Verification items for the finished model (mm, model axes). A direction names the side the tool comes from. Give positions to 0.01 mm unless a question says otherwise; leave off trailing zeros. Loops run counter-clockwise (first coordinate to the right, second up) from the corner with the lowest first, then second, coordinate; pieces in that order, holes last. Notation, with made-up numbers: (61.5, 19.25) - (92.5, 19.25) arc R29 ccw to (92.5, 39.25) - close; hole circle Ø11 at (-5, 1). An arc over 180 degrees is marked (long way). One line per item, written item: value. Start each with the question number.
1. Sectioned sample at B-B (y = 18). Record the cut outline in (x, z), plus the area to 3 significant figures.
2. Scan lines: L1, parallel to Z at x = 12, y = -33; L2, parallel to X at y = 19, z = 3.5; L3, parallel to Y at x = -8, z = -10. Record each from-to range of solid material in increasing order. Write a range as [from, to].
3. Access from +Z, -Z, +X, -X, +Y, -Y to the whole of each face (thin tool, end or side, straight path). Record for faces 5 (the cylindrical face through (9.295, 26.827, 0.35)), 6 (the flat face through (12, -25, -17)).
4. Gauge pin test, flat ends, axial feed: pin 1 (2 mm diameter, centred on x = -11.5, z = -18, fed in from -Y); pin 2 (5 mm diameter, centred on x = -10, y = 18, fed in from +Z). Record the tip position at first contact, or that the pin passes through.
5. Sectioned sample at A-A (z = 17.5). Record the cut outline in (x, y).
6. Mould release check, pull along X, two halves, no side actions. Record for faces 1 (the flat face through (22.5, -1, 0)), 2 (the flat face through (-22.5, -1, 0)), 3 (the flat face through (0, 1, 25)), 4 (the cylindrical face through (-12.488, -32.605, 15.304)): pulls with the +X half, pulls with the -X half, needs draft (parallel to the pull), parting line crosses it, or undercut.
7. Sectioned sample at C-C (z = 3). Record the cut outline in (x, y).
from build123d import *

# Parameters (mm, degrees)
SKETCH1_W           = 45
SKETCH1_H           = 80
BOSS_EXTRUDE1_DEPTH = 25
SKETCH3_R           = 3.25
CUT_EXTRUDE1_DEPTH  = 26
LPATTERN1_COUNT     = 2
LPATTERN1_PITCH     = 12
SKETCH4_R           = 2.25
CUT_EXTRUDE2_DEPTH  = 15


with BuildPart() as part:
    # Sketch1 → Boss-Extrude1 (new body, symmetric)
    with BuildSketch(Plane.XY):
        Rectangle(SKETCH1_W, SKETCH1_H)
    extrude(amount=BOSS_EXTRUDE1_DEPTH, both=True)

    # Sketch3 → Cut-Extrude1 (cut, symmetric)
    with BuildSketch(Plane.XY):
        with Locations((-10, 30)):
            Circle(SKETCH3_R)
        with Locations((10, 30)):
            Circle(SKETCH3_R)
    cut_extrude1 = extrude(amount=CUT_EXTRUDE1_DEPTH, both=True, mode=Mode.SUBTRACT)

    # LPattern1: Cut-Extrude1 ×2
    with Locations(*[(0, -i * LPATTERN1_PITCH, 0) for i in range(1, LPATTERN1_COUNT)]):
        add(cut_extrude1, mode=Mode.SUBTRACT)

    # Sketch4 → Cut-Extrude2 (cut)
    with BuildSketch(Plane.XZ.offset(40)):
        with Locations((-12, 17.5)):
            Circle(SKETCH4_R)
        with Locations((12, 17.5)):
            Circle(SKETCH4_R)
        with Locations((-12, -17.5)):
            Circle(SKETCH4_R)
        with Locations((12, -17.5)):
            Circle(SKETCH4_R)
    extrude(amount=-CUT_EXTRUDE2_DEPTH, mode=Mode.SUBTRACT)


solid = part.part
Results are:
1. outline: (-22.5, -25) - (-13.25, -25) - (-13.25, 25) - (-22.5, 25) - close; (-6.75, -25) - (6.75, -25) - (6.75, 25) - (-6.75, 25) - close; (13.25, -25) - (22.5, -25) - (22.5, 25) - (13.25, 25) - close
1. area: 1,600 mm^2
2. L1: z = [-25, -19.75], [-15.25, 15.25], [19.75, 25]
2. L2: x = [-22.5, -13.09], [-6.91, 6.91], [13.09, 22.5]
2. L3: y = [-40, 15.44], [20.56, 27.44], [32.56, 40]
3. face 5: +Z, -Z
3. face 6: -Y
4. pin 1: stops at y = -25
4. pin 2: passes through
5. outline: (-22.5, -40) - (-14.25, -40) - (-14.25, -25) - (-9.75, -25) - (-9.75, -40) - (9.75, -40) - (9.75, -25) - (14.25, -25) - (14.25, -40) - (22.5, -40) - (22.5, 40) - (-22.5, 40) - close; hole circle Ø6.5 at (-10, 18); hole circle Ø6.5 at (-10, 30); hole circle Ø6.5 at (10, 18); hole circle Ø6.5 at (10, 30)
6. face 1: pulls with the +X half
6. face 2: pulls with the -X half
6. face 3: needs draft
6. face 4: undercut
7. outline: (-22.5, -40) - (22.5, -40) - (22.5, 40) - (-22.5, 40) - close; hole circle Ø6.5 at (-10, 18); hole circle Ø6.5 at (-10, 30); hole circle Ø6.5 at (10, 18); hole circle Ø6.5 at (10, 30)
